from build123d import *

# Parameters (mm, degrees)
SKETCH1_W           = 30
SKETCH1_H           = 73
BOSS_EXTRUDE1_DEPTH = 26
SKETCH2_W           = 25
SKETCH2_H           = 16.2
CUT_EXTRUDE1_DEPTH  = 74
SKETCH3_W           = 26
SKETCH3_H           = 24
SKETCH3_H_2         = 16.23422306
CUT_EXTRUDE2_DEPTH  = 5
SKETCH5_W           = 60
SKETCH5_H           = 60
BOSS_EXTRUDE2_DEPTH = 5
FILLET1_R           = 5
SKETCH6_R           = 1.5
CUT_EXTRUDE4_DEPTH  = 5
SKETCH7_R           = 1
CUT_EXTRUDE5_DEPTH  = 4
SKETCH8_W           = 15.5
SKETCH8_H           = 5
CUT_EXTRUDE6_DEPTH  = 42
SKETCH9_W           = 5
SKETCH9_H           = 26
CUT_EXTRUDE7_DEPTH  = 73
SKETCH10_W          = 2
SKETCH10_H          = 8
SKETCH10_H_2        = 7.5
BOSS_EXTRUDE3_DEPTH = 78
SKETCH11_W          = 41.5
SKETCH11_H          = 0.7
CUT_EXTRUDE8_DEPTH  = 6
SKETCH13_W          = 0.7
SKETCH13_H          = 5
BOSS_EXTRUDE5_DEPTH = 2
SKETCH15_W          = 4
SKETCH15_H          = 16.2
BOSS_EXTRUDE6_DEPTH = 78


with BuildPart() as part:
    # Sketch1 → Boss-Extrude1 (new body)
    with BuildSketch(Plane.XY):
        Rectangle(SKETCH1_W, SKETCH1_H)
    extrude(amount=BOSS_EXTRUDE1_DEPTH)

    # Sketch2 → Cut-Extrude1 (cut, through all)
    with BuildSketch(Plane(origin=(0, 36.5, 0), x_dir=(1, 0, 0), z_dir=(0, 1, 0))):
        with Locations((-1, -13.1)):
            Rectangle(SKETCH2_W, SKETCH2_H)
    extrude(amount=-CUT_EXTRUDE1_DEPTH, mode=Mode.SUBTRACT)

    # Sketch3 → Cut-Extrude2 (cut)
    with BuildSketch(Plane.ZY.offset(15)):
        with Locations((13, 21.5)):
            Rectangle(SKETCH3_W, SKETCH3_H)
        with Locations((13, -5.5)):
            Rectangle(SKETCH3_W, SKETCH3_H)
        with Locations((13, -28.61711153)):
            Rectangle(SKETCH3_W, SKETCH3_H_2)
    extrude(amount=-CUT_EXTRUDE2_DEPTH, mode=Mode.SUBTRACT)

    # Sketch5 → Boss-Extrude2 (add)
    with BuildSketch(Plane(origin=(0, -36.5, 0), x_dir=(-1, 0, 0), z_dir=(0, -1, 0))):
        with Locations((0, -13)):
            Rectangle(SKETCH5_W, SKETCH5_H)
    extrude(amount=BOSS_EXTRUDE2_DEPTH)

    # Fillet1
    fillet1_edges = [part.edges().sort_by_distance(p)[0] for p in [
        (30, -39, -17),
        (30, -39, 43),
        (-30, -39, 43),
        (-30, -39, -17),
    ]]
    fillet(fillet1_edges, radius=FILLET1_R)

    # Sketch6 → Cut-Extrude4 (cut)
    with BuildSketch(Plane(origin=(0, -36.5, 0), x_dir=(1, 0, 0), z_dir=(0, 1, 0))):
        with Locations((-24.540514854, 12.671548216)):
            Circle(SKETCH6_R)
        with Locations((24.540514854, 12.671548216)):
            Circle(SKETCH6_R)
        with Locations((-24.540514854, -38.671548216)):
            Circle(SKETCH6_R)
        with Locations((24.540514854, -38.671548216)):
            Circle(SKETCH6_R)
    extrude(amount=-CUT_EXTRUDE4_DEPTH, mode=Mode.SUBTRACT)

    # Sketch7 → Cut-Extrude5 (cut)
    with BuildSketch(Plane(origin=(0, 0, 0), x_dir=(-1, 0, 0), z_dir=(0, 0, -1))):
        with Locations((-7, 31.5)):
            Circle(SKETCH7_R)
        with Locations((-12, 24.5)):
            Circle(SKETCH7_R)
        with Locations((-2, 24.5)):
            Circle(SKETCH7_R)
        with Locations((-7, 18.5)):
            Circle(SKETCH7_R)
    extrude(amount=-CUT_EXTRUDE5_DEPTH, mode=Mode.SUBTRACT)

    # Sketch8 → Cut-Extrude6 (cut)
    with BuildSketch(Plane.ZY.offset(30)):
        with Locations((12.75, -39)):
            Rectangle(SKETCH8_W, SKETCH8_H)
    extrude(amount=-CUT_EXTRUDE6_DEPTH, mode=Mode.SUBTRACT)

    # Sketch9 → Cut-Extrude7 (cut)
    with BuildSketch(Plane(origin=(0, 36.5, 0), x_dir=(1, 0, 0), z_dir=(0, 1, 0))):
        with Locations((-12.5, -13)):
            Rectangle(SKETCH9_W, SKETCH9_H)
    extrude(amount=-CUT_EXTRUDE7_DEPTH, mode=Mode.SUBTRACT)

    # Sketch10 → Boss-Extrude3 (add)
    with BuildSketch(Plane(origin=(0, 36.5, 0), x_dir=(1, 0, 0), z_dir=(0, 1, 0))):
        with Locations((-11, -4)):
            Rectangle(SKETCH10_W, SKETCH10_H)
        with Locations((-11, -22.25)):
            Rectangle(SKETCH10_W, SKETCH10_H_2)
    extrude(amount=-BOSS_EXTRUDE3_DEPTH)

    # Sketch11 → Cut-Extrude8 (cut, through all)
    with BuildSketch(Plane(origin=(0, -36.5, 0), x_dir=(1, 0, 0), z_dir=(0, 1, 0))):
        with Locations((-9.25, -20.85)):
            Rectangle(SKETCH11_W, SKETCH11_H)
    extrude(amount=-CUT_EXTRUDE8_DEPTH, mode=Mode.SUBTRACT)

    # Sketch13 → Boss-Extrude5 (add)
    with BuildSketch(Plane.ZY.offset(12)):
        with Locations((20.85, -39)):
            Rectangle(SKETCH13_W, SKETCH13_H)
    extrude(amount=-BOSS_EXTRUDE5_DEPTH)

    # Sketch15 → Boss-Extrude6 (add)
    with BuildSketch(Plane(origin=(0, 36.5, 0), x_dir=(1, 0, 0), z_dir=(0, 1, 0))):
        with Locations((4.4, -13.1)):
            Rectangle(SKETCH15_W, SKETCH15_H)
    extrude(amount=-BOSS_EXTRUDE6_DEPTH)


solid = part.part
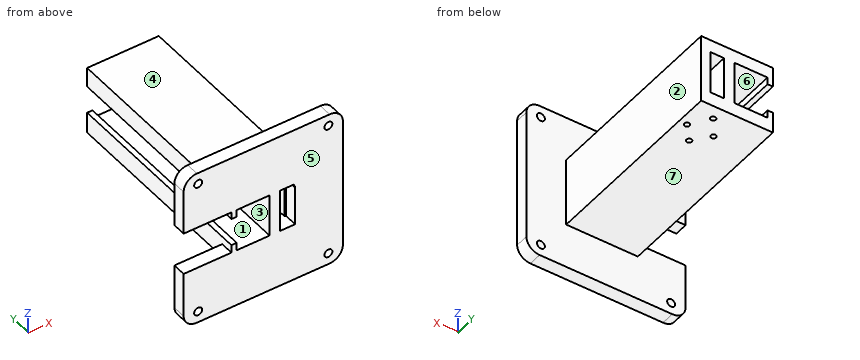
Check sheet for the modelled part. Datum: model origin and axes. Units: mm. Face numbers are marked on the shaded views. A direction names the side the tool comes from. Give positions to 0.01 mm unless a question says otherwise; leave off trailing zeros. Loops run counter-clockwise (first coordinate to the right, second up) from the corner with the lowest first, then second, coordinate; pieces in that order, holes last. Notation, with made-up numbers: M 73,-4 L 131,-4 A27 ccw 131,24 Z; hole C -3.75,-13 d10. An arc over 180 degrees is marked long. Return JSON: item names as keys, results as strings. Group by question number.
1. Cross-section at B-B on x = -16.5. Record the boundary of the cut face in (y, z).
2. Thickness scan on L1, parallel to X at y = -7, z = 16; L2, parallel to Y at x = 16.5, z = 15.5; L3, parallel to X at y = 18, z = 1. Record the ranges inside material, lowest first.
3. Cross-section at A-A on y = -15. Record the boundary of the cut face in (x, z), plus the area to 4 significant figures.
4. Mould release check, pull along X, two halves, no side actions. Record for the marked faces 1, 2, 3 and 4: released by +X, released by -X, zero draft, split by the parting line, or undercut.
5. Cross-section at C-C on z = 30.5. Record the boundary of the cut face in (x, y).
6. Cross-section at D-D on y = 18.5. Record the boundary of the cut face in (x, z).
7. Tool access check on the marked faces 5, 6 and 7. Record the directions out of +Z, -Z, +X, -X, +Y, -Y that give a thin tool (end or side, any length) a straight path to the whole face; none if there is none.
8. Go/stop test with flat-tipped pins: pin 1 (0.6 mm diameter, centred on x = 7, y = 19, fed in from -Z); pin 2 (2.5 mm diameter, centred on x = 7, y = 31.5, fed in from +Z); pin 3 (2.5 mm diameter, centred on x = 12, y = 24.5, fed in from -Z). Record where each tip stops, or that it passes through.
Return value:
{
 "1": {"outline": "M -41.5,-17 L -36.5,-17 L -36.5,5 L -41.5,5 Z; M -41.5,21.2 L -36.5,21.2 L -36.5,43 L -41.5,43 Z"},
 "2": {"L1": "2.4 to 6.4, 11.5 to 15", "L2": "-41.5 to -36.5", "L3": "-12 to 6.13, 7.87 to 15"},
 "3": {"outline": "M -12,0 L 15,0 L 15,26 L -12,26 L -12,18.5 L -10,18.5 L -10,21.2 L 2.4,21.2 L 2.4,5 L -10,5 L -10,8 L -12,8 Z; hole M 6.4,5 L 11.5,5 L 11.5,21.2 L 6.4,21.2 Z", "area": "397.5 mm^2"},
 "4": {"face 1": "undercut", "face 2": "released by +X", "face 3": "undercut", "face 4": "zero draft"},
 "5": {"outline": "M -30,-41.5 L 30,-41.5 L 30,-36.5 L -30,-36.5 Z"},
 "6": {"outline": "M -12,0 L 6,0 L 6,4 L 8,4 L 8,0 L 15,0 L 15,26 L -12,26 L -12,18.5 L -10,18.5 L -10,21.2 L 2.4,21.2 L 2.4,5 L -10,5 L -10,8 L -12,8 Z; hole M 6.4,5 L 11.5,5 L 11.5,21.2 L 6.4,21.2 Z"},
 "7": {"face 5": "+Z, -Z, +X, -X, -Y", "face 6": "+Y, -Y", "face 7": "-Z, +X, -X, +Y"},
 "8": {"pin 1": "z = 4", "pin 2": "z = 26", "pin 3": "z = 0"}
}
